The listing builds one solid part. Answer for the finished solid, in the listing's coordinates (mm). Face numbers are marked on the shaded views. Round coordinates to 2 decimals unless told otherwise and drop trailing zeros. Loops run counter-clockwise (first coordinate to the right, second up) from the corner with the lowest first, then second, coordinate; pieces in that order, holes last. Notation, with made-up numbers: (54, 84) -> (69, 84) arc R20 cw to (69, 94) -> close; hole circle Ø5 at (-37, -5.5). An arc over 180 degrees is marked (long way). Use a Markdown table: item, result. Add a question column.
Q1. Section C-C on z = 5.25 is taken. Give the vertices of the cut face in (x, y).
Q2. Section A-A on y = 0 is taken. Give the vertices of the cut face in (x, z), then the cut area to 3 significant figures.
Q3. For a pull along Y with two mould halves and no side action, classify the marked faces 1, 2, 3 and 4 as released by +Y, released by -Y, zero draft, split by the parting line, or undercut.
Q4. Consider line 1 (Y direction, x = 0, z = 4); line 2 (Y direction, x = -7.5, z = 5.5). Determine where each line is inside the solid, lowest interval first.
from build123d import *

# Parameters (mm, degrees)
CYLINDER_R     = 20
CYLINDER_DEPTH = 20
BOX_W          = 70
BOX_H          = 70
BOX_DEPTH      = 10
CHAMFER_SIZE   = 3
FILLET_R       = 3


with BuildPart() as cylinder:
    # Cylinder → Cylinder (new body)
    with BuildSketch(Plane.XY.offset(-1)):
        Circle(CYLINDER_R)
    extrude(amount=CYLINDER_DEPTH)


with BuildPart() as fillet_body:
    # Box → Box (new body)
    with BuildSketch(Plane(origin=(-35, -35, 0), x_dir=(1, 0, 0), z_dir=(0, 0, 1))):
        with Locations((35, 35)):
            Rectangle(BOX_W, BOX_H)
    extrude(amount=BOX_DEPTH)

    # Cut: cut Cylinder
    add(cylinder.part, mode=Mode.SUBTRACT)

    # Chamfer
    chamfer_edges = [fillet_body.edges().sort_by_distance(p)[0] for p in [
        (-20, 0, 10),
    ]]
    chamfer(chamfer_edges, length=CHAMFER_SIZE)

    # Fillet
    fillet_edges = [fillet_body.edges().sort_by_distance(p)[0] for p in [
        (-35, 0, 10),
        (0, 35, 10),
        (0, -35, 10),
        (35, 0, 10),
        (-35, -35, 5),
        (-35, 35, 5),
        (35, 35, 5),
        (35, -35, 5),
    ]]
    fillet(fillet_edges, radius=FILLET_R)


solid = fillet_body.part
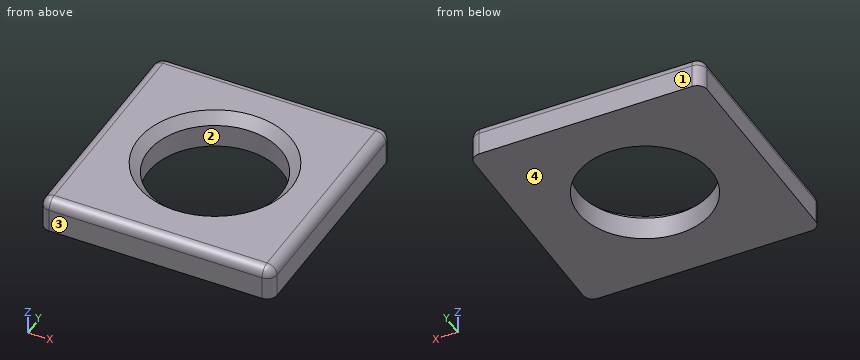
Checked values:
| question | item | result |
|---|---|---|
| 1 | outline | (-35, -32) arc R3 ccw to (-32, -35) -> (32, -35) arc R3 ccw to (35, -32) -> (35, 32) arc R3 ccw to (32, 35) -> (-32, 35) arc R3 ccw to (-35, 32) -> close; hole circle Ø40 at (0, 0) |
| 2 | outline | (-35, 0) -> (-20, 0) -> (-20, 7) -> (-23, 10) -> (-32, 10) arc R3 ccw to (-35, 7) -> close; (20, 0) -> (35, 0) -> (35, 7) arc R3 ccw to (32, 10) -> (23, 10) -> (20, 7) -> close |
| 2 | area | 287 mm2 |
| 3 | face 1 | released by +Y |
| 3 | face 2 | undercut |
| 3 | face 3 | released by -Y |
| 3 | face 4 | zero draft |
| 4 | line 1 | y = -35 to -20, 20 to 35 |
| 4 | line 2 | y = -35 to -18.54, 18.54 to 35 |
